from build123d import *

# Parameters (mm, degrees)
SKETCH1_W           = 72
SKETCH1_H           = 40
BOSS_EXTRUDE1_DEPTH = 6
SKETCH3_W           = 40
SKETCH3_H           = 15
SKETCH3_R           = 2.05
BOSS_EXTRUDE2_DEPTH = 5
FILLET2_R           = 10
FILLET1_R           = 2
BOSS_EXTRUDE3_DEPTH = 10
SKETCH6_R           = 1.55
CUT_EXTRUDE2_DEPTH  = 10
SKETCH2_R           = 2.75
CUT_EXTRUDE1_DEPTH  = 1
FILLET3_R           = 10
CUT_EXTRUDE3_START  = -7
CUT_EXTRUDE3_DEPTH  = 7
FILLET4_R           = 1.5


# Read off the part's stored shape, not the designer's step: Cut-Extrude3
with BuildPart() as part:
    # Sketch1 → Boss-Extrude1 (new body)
    with BuildSketch(Plane(origin=(0, 0, 0), x_dir=(1, 0, 0), z_dir=(0, 1, 0))):
        Rectangle(SKETCH1_W, SKETCH1_H)
    extrude(amount=BOSS_EXTRUDE1_DEPTH)

    # Sketch3 → Boss-Extrude2 (add)
    with BuildSketch(Plane(origin=(36, 0, 0), x_dir=(0, 0, -1), z_dir=(1, 0, 0))):
        with Locations((0, 7.5)):
            Rectangle(SKETCH3_W, SKETCH3_H)
        with Locations((-5, 10.5)):
            Circle(SKETCH3_R, mode=Mode.SUBTRACT)
        with Locations((5, 10.5)):
            Circle(SKETCH3_R, mode=Mode.SUBTRACT)
    boss_extrude2 = extrude(amount=BOSS_EXTRUDE2_DEPTH)

    # Mirror1: Boss-Extrude2 across plane
    add(boss_extrude2.mirror(Plane.ZY))

    # Fillet2
    fillet2_edges = [part.edges().sort_by_distance(p)[0] for p in [
        (38.5, 15, -20),
    ]]
    fillet(fillet2_edges, radius=FILLET2_R)

    # Fillet1
    fillet1_edges = [part.edges().sort_by_distance(p)[0] for p in [
        (41, 0, 0),
        (-41, 0, 0),
    ]]
    fillet(fillet1_edges, radius=FILLET1_R)

    # Sketch5 → Boss-Extrude3 (add)
    with BuildSketch(Plane.XY.offset(20)):
        with BuildLine():
            Line((-41, 15), (-41, 2))
            ThreePointArc((-41, 2), (-40.414213562, 0.585786438), (-39, 0))
            Line((-39, 0), (39, 0))
            ThreePointArc((39, 0), (40.414213562, 0.585786438), (41, 2))
            Line((41, 2), (41, 15))
            Line((41, 15), (36, 15))
            Line((36, 15), (36, 6))
            Line((36, 6), (-36, 6))
            Line((-36, 6), (-36, 15))
            Line((-36, 15), (-41, 15))
        make_face()
    extrude(amount=BOSS_EXTRUDE3_DEPTH)

    # Sketch6 → Cut-Extrude2 (cut)
    with BuildSketch(Plane.XZ):
        with Locations(Location((24, 24, 0), (0, 0, 270))):
            Circle(SKETCH6_R)
        with Locations(Location((24, -8, 0), (0, 0, 270))):
            Circle(SKETCH6_R)
        with Locations(Location((-24, 24, 0), (0, 0, 270))):
            Circle(SKETCH6_R)
        with Locations(Location((-24, -8, 0), (0, 0, 270))):
            Circle(SKETCH6_R)
    extrude(amount=-CUT_EXTRUDE2_DEPTH, mode=Mode.SUBTRACT)

    # Sketch2 → Cut-Extrude1 (cut)
    with BuildSketch(Plane(origin=(0, 6, 0), x_dir=(1, 0, 0), z_dir=(0, 1, 0))):
        with Locations(Location((-24, 8, 0), (0, 0, 270))):
            Circle(SKETCH2_R)
        with Locations(Location((-24, -24, 0), (0, 0, 270))):
            Circle(SKETCH2_R)
        with Locations(Location((24, -24, 0), (0, 0, 270))):
            Circle(SKETCH2_R)
        with Locations(Location((24, 8, 0), (0, 0, 270))):
            Circle(SKETCH2_R)
    extrude(amount=-CUT_EXTRUDE1_DEPTH, mode=Mode.SUBTRACT)

    # Fillet3
    fillet3_edges = [part.edges().sort_by_distance(p)[0] for p in [
        (-38.5, 15, 30),
    ]]
    fillet(fillet3_edges, radius=FILLET3_R)

    # Cut-Extrude3 outline → Cut-Extrude3 (cut)
    with BuildSketch(Plane.ZY.offset(41).offset(CUT_EXTRUDE3_START)):
        with BuildLine():
            Line((12.245425122, 15), (18.589156814, 11.546259248))
            ThreePointArc((18.589156814, 11.546259248), (22.57380679, 10.92053449), (26.05426141, 12.959014938))
            ThreePointArc((26.05426141, 12.959014938), (23.194514879, 14.476026313), (20, 15))
            Line((20, 15), (12.245425122, 15))
        make_face()
        Polygon((-19.449321347, 0), (-20, 5), (-20, 0), align=None)
    extrude(amount=CUT_EXTRUDE3_DEPTH, mode=Mode.SUBTRACT)

    # Fillet4
    fillet4_edges = [part.edges().sort_by_distance(p)[0] for p in [
        (-38.5, 12.959014938, 26.05426141),
    ]]
    fillet(fillet4_edges, radius=FILLET4_R)


solid = part.part
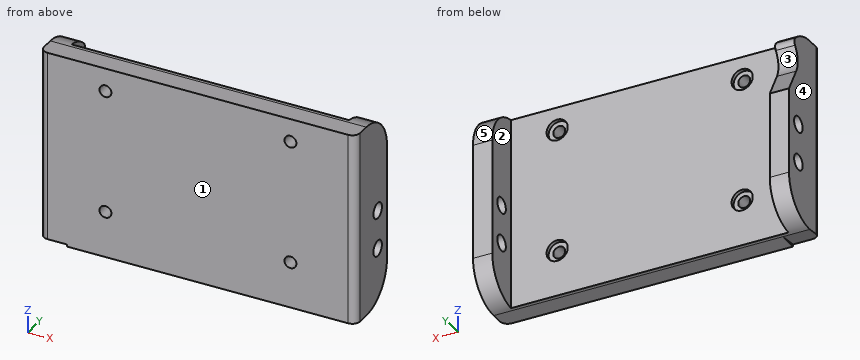
The listing builds one solid part. Answer for the finished solid, in the listing's coordinates (mm). Face numbers are marked on the shaded views. A direction names the side the tool comes from. Give positions to 0.01 mm unless a question says otherwise; leave off trailing zeros. Write each loop counter-clockwise with the first axis right and the second up, starting at its lowest first coordinate (ties: lowest second). Pieces come first, ordered by that corner, then holes.
1) For a pull along Z with two mould halves and no side action, classify the marked faces 3, 4 and 5 as pulls with the +Z half, pulls with the -Z half, needs draft (parallel to the pull), parting line crosses it, or undercut.
2) A tool of negligible diameter and unlimited length cuts with its end or side. For the marked faces 1 and 2, from which of +Z, -Z, +X, -X, +Y, -Y can it reach the whole face along a straight path? Write none if from no direction.
3) Find the intervals of material crossed by L1, parallel to X at y = 5.6, z = -8; L2, parallel to X at y = 2.8, z = -8; L3, parallel to X at y = 11, z = -12.5, in increasing order.
4) Section A-A (z = 5) is taken. Write down the section's boundary in (x, y).
5) Section D-D (z = -0.5) is taken. Write down the section's boundary in (x, y).
6) Given P1, Ø3.5, axis at x = -24, z = -8, coming from the +Y side; P2, Ø4.5, axis at x = 25, z = -9, coming from the +Y side; P3, Ø1.5, axis at x = 28.5, y = 6.5, coming from the -Z side, each flat-ended and moving along its own axis, determine where each tip first touches the part or whether it passes through.
7) Section B-B (x = -24) is taken. Write down the section's boundary in (y, z), and give its area (3 significant figures).
8) Section C-C (y = 14) is taken. Write down the section's boundary in (x, z).
Response:
1. face 3: undercut
1. face 4: needs draft
1. face 5: pulls with the +Z half
2. face 1: +Z, -Z, +X, -X, -Y
2. face 2: +Z, -Z, +Y
3. L1: x = -41 to -26.75, -21.25 to 21.25, 26.75 to 41
3. L2: x = -41 to -25.55, -22.45 to 22.45, 25.55 to 41
3. L3: x = -41 to -36, 36 to 41
4. outline: (-41, 2) arc R2 ccw to (-39, 0) - (39, 0) arc R2 ccw to (41, 2) - (41, 8.45) - (36, 8.45) - (36, 6) - (-36, 6) - (-36, 8.45) - (-41, 8.45) - close; (-41, 12.55) - (-36, 12.55) - (-36, 15) - (-41, 15) - close; (36, 12.55) - (41, 12.55) - (41, 15) - (36, 15) - close
5. outline: (-41, 2) arc R2 ccw to (-39, 0) - (39, 0) arc R2 ccw to (41, 2) - (41, 15) - (36, 15) - (36, 6) - (-36, 6) - (-36, 15) - (-41, 15) - close
6. P1: stops at y = 5
6. P2: stops at y = 6
6. P3: stops at z = -19.97
7. outline: (0, -20) - (5, -20) arc R10 ccw to (6, -19.95) - (6, -10.75) - (5, -10.75) - (5, -9.55) - (0, -9.55) - close; (0, -6.45) - (5, -6.45) - (5, -5.25) - (6, -5.25) - (6, 21.25) - (5, 21.25) - (5, 22.45) - (0, 22.45) - close; (0, 25.55) - (5, 25.55) - (5, 26.75) - (6, 26.75) - (6, 29.95) arc R10 ccw to (5, 30) - (0, 30) - close
7. area: 258 mm2
8. outline: (-41, -14.36) - (-36, -14.36) - (-36, 14.08) - (-41, 14.08) - close; (36, -14.36) - (41, -14.36) - (41, 24.36) - (36, 24.36) - close
